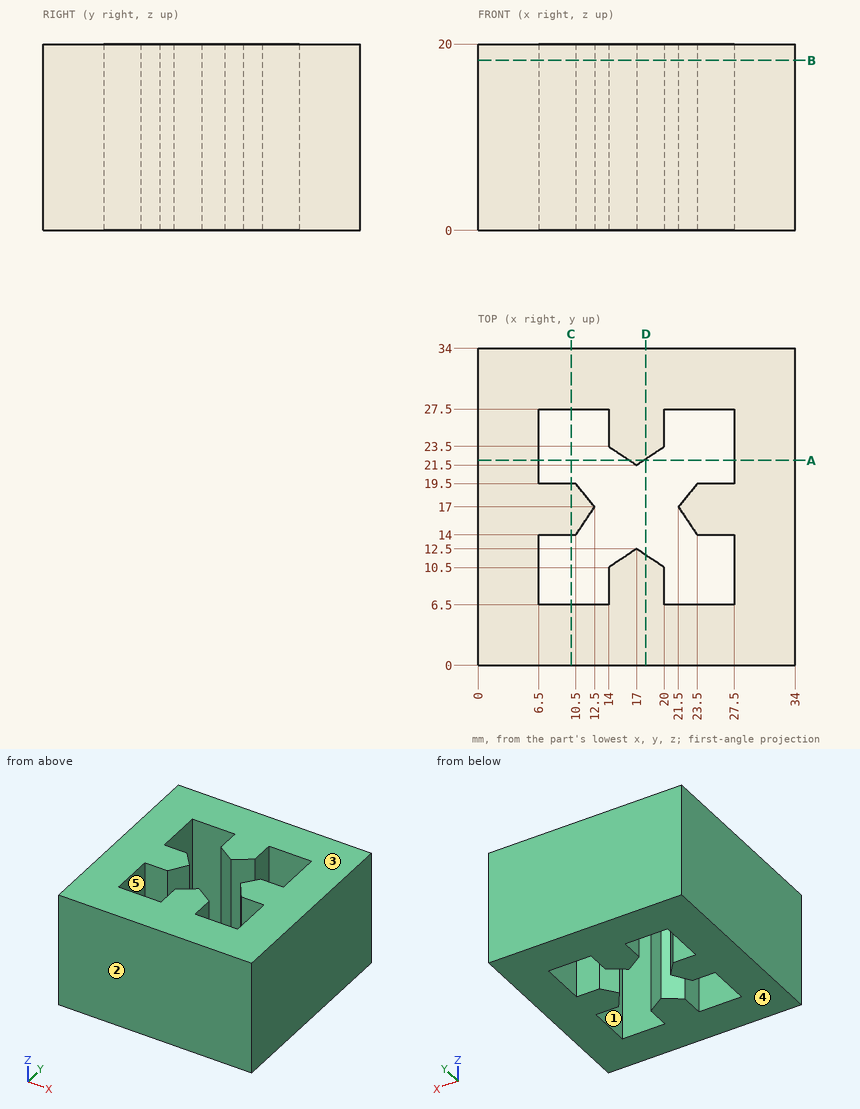
Design review of the part shown in the three views and the two pictorial views. Dimensions are in mm from the part's minimum x, y and z. A direction names the side the tool comes from. Give positions to 0.01 mm unless a question says otherwise; leave off trailing zeros. Order: outer loops, then holes, each group sorted by start corner. A loop starts at its lowest first (then second) coordinate and runs counter-clockwise, first axis right, second up. Notation, with made-up numbers: (0.5, 14.5) -> (23.5, 14.5) arc R33 cw to (23.5, 49.5) -> close; hole circle Ø9 at (48.5, 84). An arc over 180 degrees is marked (long way). Write each question's results on one line, items separated by ' | '. Start each with the question number.
Q1. Wall thickness on L1, parallel to Y at x = 24, z = 16.25; L2, parallel to X at y = 27, z = 15.75; L3, parallel to Y at x = 13.5, z = 11.5: over which ranges is each line inside the solid? List them lowest first. Write a range as from..to.
Q2. Add section D-D on x = 18. Give the boundary of the cut face in (y, z), and give its area (3 significant figures).
Q3. Add section B-B on z = 18.25. Give the boundary of the cut face in (x, y).
Q4. Machinability: for the marked faces 4 and 5, which of the approach directions +Z, -Z, +X, -X, +Y, -Y give a long, thin tool a straight path to every point of the face, cutting with its end or side? Answer none if there is none.
Q5. Add section C-C on x = 10. Give the boundary of the cut face in (y, z).
Q6. Add section A-A on y = 22. Give the boundary of the cut face in (x, z), and give its area (3 significant figures).
Q7. Mouldability with a two-part tool opening along Y and no side actions: class the marked faces 1, 2 and 3 as +Y half, -Y half, draft (parallel to the pull), parting line (faces both ways), or undercut.
Found:
1) L1: y = 0..6.5, 14..19.5, 27.5..34 | L2: x = 0..6.5, 14..20, 27.5..34 | L3: y = 0..6.5, 27.5..34
2) outline: (0, 0) -> (11.83, 0) -> (11.83, 20) -> (0, 20) -> close; (22.17, 0) -> (34, 0) -> (34, 20) -> (22.17, 20) -> close | area: 473 mm2
3) outline: (0, 0) -> (34, 0) -> (34, 34) -> (0, 34) -> close; hole (6.5, 6.5) -> (14, 6.5) -> (14, 10.5) -> (17, 12.5) -> (20, 10.5) -> (20, 6.5) -> (27.5, 6.5) -> (27.5, 14) -> (23.5, 14) -> (21.5, 17) -> (23.5, 19.5) -> (27.5, 19.5) -> (27.5, 27.5) -> (20, 27.5) -> (20, 23.5) -> (17, 21.5) -> (14, 23.5) -> (14, 27.5) -> (6.5, 27.5) -> (6.5, 19.5) -> (10.5, 19.5) -> (12.5, 17) -> (10.5, 14) -> (6.5, 14) -> close
4) face 4: -Z, +X, -X, +Y, -Y | face 5: +Z, -Z
5) outline: (0, 0) -> (6.5, 0) -> (6.5, 20) -> (0, 20) -> close; (14, 0) -> (19.5, 0) -> (19.5, 20) -> (14, 20) -> close; (27.5, 0) -> (34, 0) -> (34, 20) -> (27.5, 20) -> close
6) outline: (0, 0) -> (6.5, 0) -> (6.5, 20) -> (0, 20) -> close; (16.25, 0) -> (17.75, 0) -> (17.75, 20) -> (16.25, 20) -> close; (27.5, 0) -> (34, 0) -> (34, 20) -> (27.5, 20) -> close | area: 290 mm2
7) face 1: undercut | face 2: -Y half | face 3: draft
